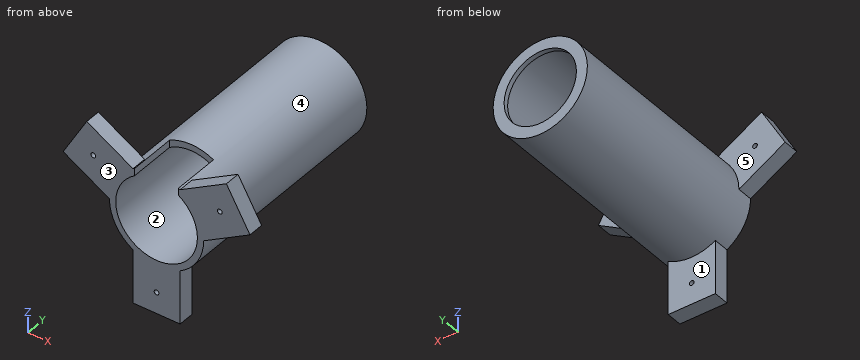
from build123d import *

# Parameters (mm, degrees)
SKETCH1_R           = 15
SKETCH1_R_2         = 13
BOSS_EXTRUDE1_DEPTH = 68.58
SKETCH2_R           = 15
SKETCH2_R_2         = 11.5
BOSS_EXTRUDE2_DEPTH = 1.5
SKETCH3_W           = 14
SKETCH3_H           = 15.591369762
CUT_EXTRUDE1_DEPTH  = 15
SKETCH4_R           = 0.75
BOSS_EXTRUDE3_DEPTH = 5
CIRPATTERN1_COUNT   = 3


with BuildPart() as part:
    # Sketch1 → Boss-Extrude1 (new body)
    with BuildSketch(Plane(origin=(0, 0, 0), x_dir=(1, 0, 0), z_dir=(0, 1, 0))):
        with Locations(Location((0, 0, 0), (0, 0, 270))):
            Circle(SKETCH1_R)
        with Locations(Location((0, 0, 0), (0, 0, 270))):
            Circle(SKETCH1_R_2, mode=Mode.SUBTRACT)
    extrude(amount=BOSS_EXTRUDE1_DEPTH)

    # Sketch2 → Boss-Extrude2 (add)
    with BuildSketch(Plane(origin=(0, 68.58, 0), x_dir=(1, 0, 0), z_dir=(0, 1, 0))):
        with Locations(Location((0, 0, 0), (0, 0, 270))):
            Circle(SKETCH2_R)
        with Locations(Location((0, 0, 0), (0, 0, 270))):
            Circle(SKETCH2_R_2, mode=Mode.SUBTRACT)
    extrude(amount=BOSS_EXTRUDE2_DEPTH)

    # Sketch3 → Cut-Extrude1 (cut)
    with BuildSketch(Plane.XZ):
        with Locations((0, 7.795684881)):
            Rectangle(SKETCH3_W, SKETCH3_H)
    extrude(amount=-CUT_EXTRUDE1_DEPTH, mode=Mode.SUBTRACT)

    # Sketch4 → Boss-Extrude3 (add)
    with BuildSketch(Plane.XZ):
        with BuildLine():
            Line((-7.5, -12.990381057), (-7.5, -30))
            Line((-7.5, -30), (7.5, -30))
            Line((7.5, -30), (7.5, -12.990381057))
            ThreePointArc((7.5, -12.990381057), (0, -15), (-7.5, -12.990381057))
        make_face()
        with Locations(Location((0, -23.25, 0), (0, 0, 270))):
            Circle(SKETCH4_R, mode=Mode.SUBTRACT)
    boss_extrude3 = extrude(amount=-BOSS_EXTRUDE3_DEPTH)

    # CirPattern1: Boss-Extrude3 ×3 about axis
    cirpattern1_axis = Axis((0, 0, 0), (0, 1, 0))
    for i in range(1, CIRPATTERN1_COUNT):
        add(boss_extrude3.rotate(cirpattern1_axis, i * 360 / CIRPATTERN1_COUNT))


solid = part.part
Can you work these out from the model? Positions are in its coordinate system, mm. Face numbers are marked on the shaded views. A direction names the side the tool comes from. Coordinates: 2 decimals unless noted, no trailing zeros. Write each loop counter-clockwise with the first axis right and the second up, starting at its lowest first coordinate (ties: lowest second). Pieces come first, ordered by that corner, then holes. Notation, with made-up numbers: M 64,89 L 71,89 A24 cw 71,113 Z; hole C -11,57 d9. An arc over 180 degrees is marked long. Use one line per item in the form item = value.
Q1. We'd pull the mould along X, two halves only. Please class the marked faces 1 and 2: +X half, -X half, draft (parallel to the pull), parting line (faces both ways), or undercut.
Model answer:
face_1 = draft
face_2 = undercut
Q2. For the marked faces 3, 4 and 5, which set-ups out of +Z, -Z, +X, -X, +Y, -Y let a thin tool reach every point of the face, with its end or its side?
Model answer:
face_3 = +Z, -Z, +X, -X, -Y
face_4 = +Y
face_5 = +Z, -X, +Y
Q3. If we section it at C-C (y = 6.5): Write out the boundary of the cut face in (x, z).
Model answer:
outline = M -7,10.95 L -7,13.27 A15 ccw long 7,13.27 L 7,10.95 A13 cw long Z
Q4. If we section it at A-A (z = -5): Write out the boundary of the cut face in (x, y), then the cut area to 3 significant figures.
Model answer:
outline = M -14.14,0 L -12,0 L -12,68.58 L -10.36,68.58 L -10.36,70.08 L -14.14,70.08 Z; M 10.36,68.58 L 12,68.58 L 12,0 L 14.14,0 L 14.14,70.08 L 10.36,70.08 Z
area = 305 mm^2
Q5. If we section it at B-B (x = -2): Write out the boundary of the cut face in (y, z).
Model answer:
outline = M 0,-30 L 5,-30 L 5,-14.87 L 70.08,-14.87 L 70.08,-11.32 L 68.58,-11.32 L 68.58,-12.85 L 0,-12.85 Z; M 15,12.85 L 68.58,12.85 L 68.58,11.32 L 70.08,11.32 L 70.08,14.87 L 15,14.87 Z
Q6. I need wall thicknesses on line 1 along X through (y, z) = (69, 0); line 2 along X through (y, z) = (44.5, 0); line 3 along Y through (x, z) = (9, 8). Which ranges of each line are inside material? Lowest first, please. Write a range as from..to.
Model answer:
line_1 = -15..-11.5, 11.5..15
line_2 = -15..-13, 13..15
line_3 = 68.58..70.08
Q7. If we section it at D-D (y = 47.5): Write out the boundary of the cut face in (x, z), then the cut area to 3 significant figures.
Model answer:
outline = C 0,0 d30; hole C 0,0 d26
area = 176 mm^2
Q8. For P1, Ø3, axis at x = 15, y = 55.5, coming from the -Z side; P2, Ø2, axis at x = -2.5, z = 14, coming from the -Y side; P3, Ø2, axis at y = 55.5, z = 13, coming from the -X side; P4, Ø8, axis at x = -11, z = -1.5, coming from the +Y side, each with a flat end and sliding along its axis, tell me the tip position at first contact or that it passes through.
Model answer:
P1 = -6.54
P2 = 15
P3 = -9
P4 = 70.08
